Read the model definition and answer for the solid it produces. Units are mm, in the model's axes. Coordinates: 2 decimals unless noted, no trailing zeros. Write each loop counter-clockwise with the first axis right and the second up, starting at its lowest first coordinate (ties: lowest second). Pieces come first, ordered by that corner, then holes. Notation, with made-up numbers: M 58.25,48.25 L 102.25,48.25 A4 ccw 102.25,54.25 Z; hole C -38.75,-19.5 d9. An arc over 180 degrees is marked long. Use a Markdown table: item, result. Add a question column.
from build123d import *

# Parameters (mm, degrees)
CROQUIS1_W              = 39.5
CROQUIS1_H              = 80
SALIENTE_EXTRUIR1_DEPTH = 10
CROQUIS2_R              = 4
CORTAR_EXTRUIR1_DEPTH   = 82
CROQUIS3_R              = 1.6
CORTAR_EXTRUIR2_DEPTH   = 11


with BuildPart() as part:
    # Croquis1 → Saliente-Extruir1 (new body)
    with BuildSketch(Plane(origin=(0, 0, 0), x_dir=(1, 0, 0), z_dir=(0, 1, 0))):
        Rectangle(CROQUIS1_W, CROQUIS1_H)
    extrude(amount=SALIENTE_EXTRUIR1_DEPTH)

    # Croquis2 → Cortar-Extruir1 (cut)
    with BuildSketch(Plane.XY.offset(40)):
        with Locations((-10, -1)):
            Circle(CROQUIS2_R)
        with Locations((10, -1)):
            Circle(CROQUIS2_R)
    extrude(amount=-CORTAR_EXTRUIR1_DEPTH, mode=Mode.SUBTRACT)

    # Croquis3 → Cortar-Extruir2 (cut)
    with BuildSketch(Plane(origin=(0, 10, 0), x_dir=(1, 0, 0), z_dir=(0, 1, 0))):
        with Locations(Location((-16.875, 30, 0), (0, 0, 270))):
            Circle(CROQUIS3_R)
        with Locations(Location((0, 30, 0), (0, 0, 270))):
            Circle(CROQUIS3_R)
        with Locations(Location((16.875, 30, 0), (0, 0, 270))):
            Circle(CROQUIS3_R)
        with Locations(Location((-16.875, -30, 0), (0, 0, 270))):
            Circle(CROQUIS3_R)
        with Locations(Location((0, -30, 0), (0, 0, 270))):
            Circle(CROQUIS3_R)
        with Locations(Location((16.875, -30, 0), (0, 0, 270))):
            Circle(CROQUIS3_R)
    extrude(amount=-CORTAR_EXTRUIR2_DEPTH, mode=Mode.SUBTRACT)


solid = part.part
Item 1: Determine the mould class of faces 1 (the flat face through (0, 5, -40)), 2 (the cylindrical face through (17.956, 5.07, -31.179)), 3 (the cylindrical face through (-15.794, 5.07, 28.821)), 4 (the flat face through (0, 5, 40)) for opening direction Z: pulls with the +Z half, pulls with the -Z half, needs draft (parallel to the pull), parting line crosses it, or undercut.
Item 2: Find section D-D on y = 6.25. Give the vertices of the cut face in (x, z) (3 decimals).
Item 3: Find section C-C on y = 1. Count the separate pieces of the cut face and the enclosed holes in it, then the cut area to 3 significant figures.
Item 4: Consider probe 1 along X at (y, z) = (5.25, 30) (3 decimals); probe 2 along Z at (x, y) = (16.5, 9.5); probe 3 along Z at (x, y) = (-17.5, 7.5). Determine where each line is inside the solid, lowest interval first.
Item 5: Find section A-A on x = 0. Give the vertices of the cut face in (y, z), then the cut area to 3 significant figures.
Item 6: Find section B-B on z = 30. Give the vertices of the cut face in (x, y) (3 decimals), then the cut area to 3 significant figures.
Geometry says:
| question | item | result |
|---|---|---|
| 1 | face 1 | pulls with the -Z half |
| 1 | face 2 | undercut |
| 1 | face 3 | undercut |
| 1 | face 4 | pulls with the +Z half |
| 2 | outline | M -19.75,-40 L 19.75,-40 L 19.75,40 L -19.75,40 Z; hole C -16.875,-30 d3.2; hole C -16.875,30 d3.2; hole C 0,-30 d3.2; hole C 0,30 d3.2; hole C 16.875,-30 d3.2; hole C 16.875,30 d3.2 |
| 3 | separate pieces | 3 |
| 3 | enclosed holes | 6 |
| 3 | area | 2,000 mm2 |
| 4 | probe 1 | x = -19.75 to -18.475, -15.275 to -1.6, 1.6 to 15.275, 18.475 to 19.75 |
| 4 | probe 2 | z = -40 to -31.56, -28.44 to 28.44, 31.56 to 40 |
| 4 | probe 3 | z = -40 to -31.47, -28.53 to 28.53, 31.47 to 40 |
| 5 | outline | M 0,-40 L 10,-40 L 10,-31.6 L 0,-31.6 Z; M 0,-28.4 L 10,-28.4 L 10,28.4 L 0,28.4 Z; M 0,31.6 L 10,31.6 L 10,40 L 0,40 Z |
| 5 | area | 736 mm2 |
| 6 | outline | M -19.75,0 L -18.475,0 L -18.475,10 L -19.75,10 Z; M -15.275,0 L -13.873,0 A4 cw -6.127,0 L -1.6,0 L -1.6,10 L -15.275,10 Z; M 1.6,0 L 6.127,0 A4 cw 13.873,0 L 15.275,0 L 15.275,10 L 1.6,10 Z; M 18.475,0 L 19.75,0 L 19.75,10 L 18.475,10 Z |
| 6 | area | 265 mm2 |
